from build123d import *

# Parameters (mm, degrees)
SKETCH1_W           = 89
SKETCH1_H           = 134
SKETCH1_R           = 1.5
SKETCH1_R_2         = 1.55
SKETCH1_W_2         = 2.2
SKETCH1_H_2         = 5
SKETCH1_W_3         = 5
SKETCH1_H_3         = 2.2
BOSS_EXTRUDE1_DEPTH = 2
FILLET1_R           = 1


with BuildPart() as part:
    # Sketch1 → Boss-Extrude1 (new body)
    with BuildSketch(Plane.XY):
        Rectangle(SKETCH1_W, SKETCH1_H)
        with Locations((-32.88, 56)):
            Circle(SKETCH1_R, mode=Mode.SUBTRACT)
        with Locations((-8.38, 56)):
            Circle(SKETCH1_R, mode=Mode.SUBTRACT)
        with Locations((-32.88, 9.5)):
            Circle(SKETCH1_R, mode=Mode.SUBTRACT)
        with Locations((-8.38, 9.5)):
            Circle(SKETCH1_R, mode=Mode.SUBTRACT)
        with Locations((1.54, 55.08)):
            Circle(SKETCH1_R, mode=Mode.SUBTRACT)
        with Locations((32.58, 55.08)):
            Circle(SKETCH1_R, mode=Mode.SUBTRACT)
        with Locations((1.54, 10.38)):
            Circle(SKETCH1_R, mode=Mode.SUBTRACT)
        with Locations((32.58, 10.38)):
            Circle(SKETCH1_R, mode=Mode.SUBTRACT)
        with Locations((-41.4, 63.4)):
            Circle(SKETCH1_R_2, mode=Mode.SUBTRACT)
        with Locations(Location((-41.4, -63.4, 0), (0, 0, 180))):
            Circle(SKETCH1_R_2, mode=Mode.SUBTRACT)
        with Locations((41.4, -63.4)):
            Circle(SKETCH1_R_2, mode=Mode.SUBTRACT)
        with Locations(Location((41.4, 63.4, 0), (0, 0, 180))):
            Circle(SKETCH1_R_2, mode=Mode.SUBTRACT)
        with Locations((-41.4, 0)):
            Rectangle(SKETCH1_W_2, SKETCH1_H_2, mode=Mode.SUBTRACT)
        with Locations((-41.4, -54.4)):
            Rectangle(SKETCH1_W_2, SKETCH1_H_2, mode=Mode.SUBTRACT)
        with Locations((-41.4, 54.4)):
            Rectangle(SKETCH1_W_2, SKETCH1_H_2, mode=Mode.SUBTRACT)
        with Locations((41.4, 54.4)):
            Rectangle(SKETCH1_W_2, SKETCH1_H_2, mode=Mode.SUBTRACT)
        with Locations((41.4, -54.4)):
            Rectangle(SKETCH1_W_2, SKETCH1_H_2, mode=Mode.SUBTRACT)
        with Locations((41.4, 0)):
            Rectangle(SKETCH1_W_2, SKETCH1_H_2, mode=Mode.SUBTRACT)
        with Locations((32.4, 63.4)):
            Rectangle(SKETCH1_W_3, SKETCH1_H_3, mode=Mode.SUBTRACT)
        with Locations((-32.4, 63.4)):
            Rectangle(SKETCH1_W_3, SKETCH1_H_3, mode=Mode.SUBTRACT)
        with Locations((32.4, -63.4)):
            Rectangle(SKETCH1_W_3, SKETCH1_H_3, mode=Mode.SUBTRACT)
        with Locations((-32.4, -63.4)):
            Rectangle(SKETCH1_W_3, SKETCH1_H_3, mode=Mode.SUBTRACT)
    extrude(amount=BOSS_EXTRUDE1_DEPTH)

    # Fillet1
    fillet1_edges = [part.edges().sort_by_distance(p)[0] for p in [
        (44.5, -67, 1),
        (-44.5, -67, 1),
        (-44.5, 67, 1),
        (44.5, 67, 1),
    ]]
    fillet(fillet1_edges, radius=FILLET1_R)


solid = part.part
The model under review builds one solid part; all positions refer to its coordinate system, in mm. Round coordinates to 2 decimals unless told otherwise and drop trailing zeros. Write each loop counter-clockwise with the first axis right and the second up, starting at its lowest first coordinate (ties: lowest second). Pieces come first, ordered by that corner, then holes. Notation, with made-up numbers: M 50.5,49.5 L 93.5,49.5 A26 cw 93.5,69.5 Z; hole C -11,82 d9. An arc over 180 degrees is marked long. Use a Markdown table: item, result. Add a question column.
Q1. Insertion check: pin 1 (1.9 mm diameter, centred on x = 41.4, y = 63.4, fed in from -Z); pin 2 (3 mm diameter, centred on x = 12, y = 37, fed in from -Z). Each pin has a flat end and moves straight along its axis. Give the tip position at first contact, or say it passes through.
Q2. To check wall thickness, follow line 1 (Y direction, x = 1.54, z = 0.9); line 2 (Y direction, x = -8.5, z = 1.2); line 3 (Y direction, x = -41.4, z = 0.7). State the ranges of each line that lie inside material, in increasing order.
Q3. The part is to be moulded in two halves that separate along Y. For faces 1 (the face through (-9.57, 55.09, 0.99)), 2 (the face through (-41.064, -61.887, 0.986)), 3 (the face through (-1, 1, 2)), say which applies: pulls with the +Y half, pulls with the -Y half, needs draft (parallel to the pull), parting line crosses it, or undercut.
Q4. We need section A-A, the plane x = 32.58. State the section outline as (y, z) points, plus the area to 3 significant figures.
Q5. We need section B-B, the plane x = 1.54. State the section outline as (y, z) points, plus the area to 3 significant figures.
Q6. We need section C-C, the plane z = 1.65. Count the separate pieces of the cut face and the enclosed holes in it, plus the area to 3 significant figures.
Findings below:
| question | item | result |
|---|---|---|
| 1 | pin 1 | passes through |
| 1 | pin 2 | stops at z = 0 |
| 2 | line 1 | y = -67 to 8.88, 11.88 to 53.58, 56.58 to 67 |
| 2 | line 2 | y = -67 to 8, 11 to 54.5, 57.5 to 67 |
| 2 | line 3 | y = -67 to -64.95, -61.85 to -56.9, -51.9 to -2.5, 2.5 to 51.9, 56.9 to 61.85, 64.95 to 67 |
| 3 | face 1 | undercut |
| 3 | face 2 | undercut |
| 3 | face 3 | needs draft |
| 4 | outline | M -67,0 L -64.5,0 L -64.5,2 L -67,2 Z; M -62.3,0 L 8.88,0 L 8.88,2 L -62.3,2 Z; M 11.88,0 L 53.58,0 L 53.58,2 L 11.88,2 Z; M 56.58,0 L 62.3,0 L 62.3,2 L 56.58,2 Z; M 64.5,0 L 67,0 L 67,2 L 64.5,2 Z |
| 4 | area | 247 mm² |
| 5 | outline | M -67,0 L 8.88,0 L 8.88,2 L -67,2 Z; M 11.88,0 L 53.58,0 L 53.58,2 L 11.88,2 Z; M 56.58,0 L 67,0 L 67,2 L 56.58,2 Z |
| 5 | area | 256 mm² |
| 6 | separate pieces | 1 |
| 6 | enclosed holes | 22 |
| 6 | area | 11,700 mm² |
